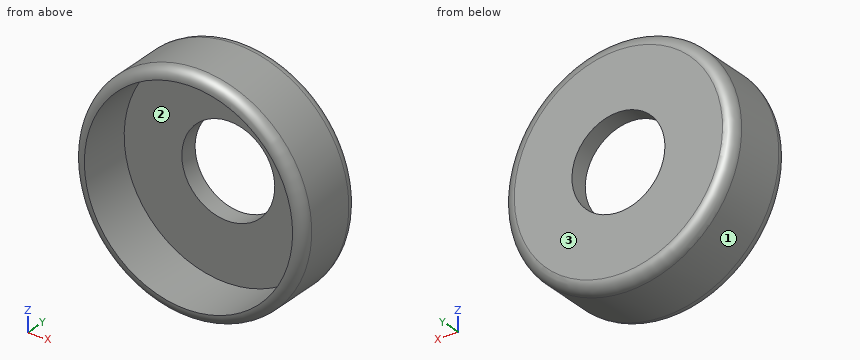
```python
from build123d import *

# Parameters (mm, degrees)
SKETCH1_R               = 31
BOSS_EXTRUDE1_DEPTH     = 20
FILLET1_R               = 3
SKETCH2_R               = 28
CUT_EXTRUDE1_DEPTH      = 15
CUT_EXTRUDE2_DEPTH      = 49.187135341
CUT_EXTRUDE2_DEPTH_BACK = 49.187135341
SKETCH3_R               = 12.5


with BuildPart() as part:
    # Sketch1 → Boss-Extrude1 (new body)
    with BuildSketch(Plane(origin=(0, 0, 0), x_dir=(1, 0, 0), z_dir=(0, 1, 0))):
        with Locations(Location((0, 0, 0), (0, 0, 270))):
            Circle(SKETCH1_R)
    extrude(amount=BOSS_EXTRUDE1_DEPTH)

    # Fillet1
    fillet1_edges = [part.edges().sort_by_distance(p)[0] for p in [
        (0, 0, -31),
        (0, 20, -31),
    ]]
    fillet(fillet1_edges, radius=FILLET1_R)

    # Sketch2 → Cut-Extrude1 (cut)
    with BuildSketch(Plane.XZ):
        with Locations(Location((0, 0, 0), (0, 0, 270))):
            Circle(SKETCH2_R)
    extrude(amount=-CUT_EXTRUDE1_DEPTH, mode=Mode.SUBTRACT)

    # Sketch3 → Cut-Extrude2 (cut, two sides: drawn at the far end of the back side and taken through both)
    with BuildSketch(Plane(origin=(0, 20, 0), x_dir=(1, 0, 0), z_dir=(0, 1, 0)).offset(-CUT_EXTRUDE2_DEPTH_BACK)):
        with Locations(Location((0, 0, 0), (0, 0, 270))):
            Circle(SKETCH3_R)
    extrude(amount=CUT_EXTRUDE2_DEPTH + CUT_EXTRUDE2_DEPTH_BACK, mode=Mode.SUBTRACT)


solid = part.part
```
Geometry: final body of the model. Coordinates: model frame, mm. Face numbers are marked on the shaded views. Coordinates: 2 decimals unless noted, no trailing zeros. Order: outer loops, then holes, each group sorted by start corner. A loop starts at its lowest first (then second) coordinate and runs counter-clockwise, first axis right, second up. Notation, with made-up numbers: M -7.75,50.5 L 18.25,50.5 A18 cw 18.25,73.5 Z; hole C 70,69 d11. An arc over 180 degrees is marked long. Answer in a Markdown table with one row per item. Add a question column.
Q1. Section query D-D on y = 17.75. Return the cut outline in (x, z).
Q2. Section query C-C on y = 8. Return the cut outline in (x, z), and give its area (3 significant figures).
Q3. Contact query for flat-ended pins moving along their axis: P1, Ø6, axis at y = 9.5, z = 0, coming from the +X side; P2, Ø20, axis at x = 0, z = 0, coming from the -Y side; P3, Ø2, axis at y = 4.5, z = 16.5, coming from the +X side; P4, Ø3, axis at x = 7, y = 9.5, coming from the +Z side. Output: stop coordinate, or through.
Q4. Mould query, pull axis Z, two halves, no side actions, for the marked faces 1, 2 and 3. Classes: released by +Z, released by -Z, zero draft, split by the parting line, or undercut.
Q5. Section query A-A on x = 0. Return the cut outline in (y, z), and give its area (3 significant figures).
Q6. Line query: L1, parallel to X at y = 5.5, z = 0; L2, parallel to X at y = 15.25, z = -0.5; L3, parallel to Y at x = -16.5, z = 15.5. Output: solid intervals per line, ascending.
Q7. Section query B-B on z = 0. Return the cut outline in (x, y).
Completed:
| question | item | result |
|---|---|---|
| 1 | outline | C 0,0 d61.81; hole C 0,0 d25 |
| 2 | outline | C 0,0 d62; hole C 0,0 d56 |
| 2 | area | 556 mm2 |
| 3 | P1 | stops at x = 31 |
| 3 | P2 | passes through |
| 3 | P3 | stops at x = 26.85 |
| 3 | P4 | stops at z = 30.51 |
| 4 | face 1 | split by the parting line |
| 4 | face 2 | undercut |
| 4 | face 3 | zero draft |
| 5 | outline | M 0,-28 A3 ccw 3,-31 L 17,-31 A3 ccw 20,-28 L 20,-12.5 L 15,-12.5 L 15,-28 Z; M 0,28 L 15,28 L 15,12.5 L 20,12.5 L 20,28 A3 ccw 17,31 L 3,31 A3 ccw Z |
| 5 | area | 267 mm2 |
| 6 | L1 | x = -31 to -28, 28 to 31 |
| 6 | L2 | x = -31 to -12.49, 12.49 to 31 |
| 6 | L3 | y = 15 to 20 |
| 7 | outline | M -31,3 A3 ccw -28,0 L -28,15 L -12.5,15 L -12.5,20 L -28,20 A3 ccw -31,17 Z; M 12.5,15 L 28,15 L 28,0 A3 ccw 31,3 L 31,17 A3 ccw 28,20 L 12.5,20 Z |
